Source: CAD feature listing. Evaluate the final solid. Frame: model axes, mm. Give positions to 0.01 mm unless a question says otherwise; leave off trailing zeros. Write each loop counter-clockwise with the first axis right and the second up, starting at its lowest first coordinate (ties: lowest second). Pieces come first, ordered by that corner, then holes. Notation, with made-up numbers: M -10,14 L 27,14 A24 ccw 27,33 Z; hole C 73.5,67.5 d11. An arc over 180 degrees is marked long. Use CSV: the item, a comma, the result in double quotes. Start each with the question number.
from build123d import *

# Parameters (mm, degrees)
SKETCH1_R           = 6.35
BOSS_EXTRUDE1_DEPTH = 5.08


with BuildPart() as part:
    # Sketch1 → Boss-Extrude1 (new body)
    with BuildSketch(Plane.XY):
        with BuildLine():
            Line((-580.7, 12.7), (0, 12.7))
            ThreePointArc((0, 12.7), (12.7, 0), (0, -12.7))
            Line((0, -12.7), (-246.387841786, -64.485872398))
            ThreePointArc((-246.387841786, -64.485872398), (-248.101037656, -64.686359692), (-249.822299661, -64.574590494))
            Line((-249.822299661, -64.574590494), (-580.7, -12.7))
            ThreePointArc((-580.7, -12.7), (-593.4, 0), (-580.7, 12.7))
        make_face()
        Circle(SKETCH1_R, mode=Mode.SUBTRACT)
        with Locations((-580.7, 0)):
            Circle(SKETCH1_R, mode=Mode.SUBTRACT)
        with Locations((-248.347003133, -55.164536023)):
            Circle(SKETCH1_R, mode=Mode.SUBTRACT)
    extrude(amount=-BOSS_EXTRUDE1_DEPTH)


solid = part.part
1. Section A-A on y = 0. Return loops of the section in (x, z).
2. First-contact query: pin 1 (1.5 mm diameter, centred on x = -195.5, z = -2, fed in from -Y); pin 2 (11.5 mm diameter, centred on x = 0, y = 0, fed in from +Z). Flat tips, straight axial feed; report the tip coordinate or a pass-through.
3. Section C-C on x = -266.5. Return loops of the section in (y, z).
4. Pull-direction query (X, two-part tool) for faces 1 (the cylindrical face through (-1.38, -6.2, -2.5)), 2 (the flat face through (-286, -17, 0)), 3 (the flat face through (-121.47, -38.23, -2.5)); classes: released by +X, released by -X, zero draft, split by the parting line, or undercut.
5. Line query: probe 1 along Y at (x, z) = (-580.7, -1.6); probe 2 along X at (y, z) = (2.5, -4); probe 3 along X at (y, z) = (3.5, -3.2). Output: solid intervals per line, ascending.
6. Section B-B on z = -4.15. Return loops of the section in (x, y) (3 decimals), then the cut area to 3 significant figures.
7. Section D-D on y = -31. Return loops of the section in (x, z) (3 decimals).
Resolved:
1,outline,"M -593.4,-5.08 L -587.05,-5.08 L -587.05,0 L -593.4,0 Z; M -574.35,-5.08 L -6.35,-5.08 L -6.35,0 L -574.35,0 Z; M 6.35,-5.08 L 12.7,-5.08 L 12.7,0 L 6.35,0 Z"
2,pin 1,"stops at y = -53.95"
2,pin 2,"passes through"
3,outline,"M -61.96,-5.08 L 12.7,-5.08 L 12.7,0 L -61.96,0 Z"
4,face 1,"undercut"
4,face 2,"zero draft"
4,face 3,"released by +X"
5,probe 1,"y = -12.7 to -6.35, 6.35 to 12.7"
5,probe 2,"x = -593.15 to -586.54, -574.86 to -5.84, 5.84 to 12.45"
5,probe 3,"x = -592.91 to -586, -575.4 to -5.3, 5.3 to 12.21"
6,outline,"M -580.7,-12.7 L -249.822,-64.575 A9.525 ccw -246.388,-64.486 L 0,-12.7 A12.7 ccw 0,12.7 L -580.7,12.7 A12.7 ccw Z; hole C -580.7,0 d12.7; hole C -248.347,-55.165 d12.7; hole C 0,0 d12.7"
6,area,"30,000 mm2"
7,outline,"M -463.975,-5.08 L -87.068,-5.08 L -87.068,0 L -463.975,0 Z"
